Verification items for the finished model (mm, model axes). A direction names the side the tool comes from. Round coordinates to 2 decimals unless told otherwise and drop trailing zeros. Order: outer loops, then holes, each group sorted by start corner. A loop starts at its lowest first (then second) coordinate and runs counter-clockwise, first axis right, second up. Notation, with made-up numbers: M -24,3 L 31,3 A26 cw 31,41 Z; hole C 24.5,34.25 d4. An arc over 180 degrees is marked long. One line per item, written item: value. Start each with the question number.
from build123d import *

# Parameters (mm, degrees)
F3_DEPTH     = 3.5
F4_SIZE      = 1
F5_SIZE      = 0.5
F6_T4_DEPTH  = 8.4221557451
F6_T11_DEPTH = 13.7150489639
F6_T21_DEPTH = 8.4221557451
F6_T28_DEPTH = 8.4221557451
F6_T35_DEPTH = 13.7150489639
F6_T45_DEPTH = 8.4221557451
F7_R         = 1.5
F8_R         = 1
F9_DEPTH     = 25


# Not quite as in the source:
# - a fillet or chamfer that OpenCascade refuses, or shapes differently, is made with other operations: its cross-section is extruded or revolved along the edge and cut away or added


with BuildPart() as f1:
    # F0 (on Front) → F1 (revolve)
    with BuildSketch(Plane.XZ):
        Polygon((0, 7), (0, 0), (5.5, 0), (5.5, 3.5), (6.5, 3.5), (6.5, 7), align=None)
    revolve(axis=Axis((0, 0, 5.0261294236), (0, 0, 1)))

    # F2 (on Front) → F3 (join, symmetric)
    with BuildSketch(Plane.XZ):
        Polygon((3.5, 0), (-3.5, 0), (-3.5, -2.5), (-2, -2.5), (-2, -5.5), (-3.5, -5.5), (-3.5, -7.5), (3.5, -7.5), (3.5, -5.5), (2, -5.5), (2, -2.5), (3.5, -2.5), align=None)
    extrude(amount=F3_DEPTH, both=True)

    # F4
    f4_edges = [f1.edges().sort_by_distance(p)[0] for p in [
        (3.5, -3.5, -1.25),
        (3.5, 3.5, -1.25),
        (-3.5, 3.5, -1.25),
        (-3.5, -3.5, -1.25),
        (-3.5, -3.5, -6.5),
        (3.5, -3.5, -6.5),
        (-3.5, 3.5, -6.5),
        (3.5, 3.5, -6.5),
    ]]
    chamfer(f4_edges, length=F4_SIZE)

    # F5
    f5_edges = [f1.edges().sort_by_distance(p)[0] for p in [
        (2, -3.5, -4),
        (-2, -3.5, -4),
        (-2, 3.5, -4),
        (2, 3.5, -4),
    ]]
    chamfer(f5_edges, length=F5_SIZE)

    # F6: chamfer of 1.5 on 6 edges, made by hand


with BuildPart() as f6_tool2:
    # F6_s3 → F6_t4 (new body)
    with BuildSketch(Plane(origin=(3.7276817198, -3.7276817198, 0), x_dir=(0, 0, 1), z_dir=(-0.7071067812, 0.7071067812, 0))):
        Polygon((-5.5, -5.0355339059), (-4, -3.5355339059), (-5.5, -3.5355339059), align=None)
    extrude(amount=F6_T4_DEPTH)

    split(bisect_by=Plane.XZ.offset(3.5), keep=Keep.BOTTOM)

    split(bisect_by=Plane(origin=(-3, -3, 0), x_dir=(0, 0, 1), z_dir=(0.7071067812, 0.7071067812, 0)), keep=Keep.TOP)

    split(bisect_by=Plane(origin=(1, 0, -1), x_dir=(0, 1, 0), z_dir=(0.7071067812, 0, -0.7071067812)), keep=Keep.TOP)


with BuildPart() as f1_1:
    add(f1.part)

    # F6_t1: union F6_tool2
    add(f6_tool2.part)


with BuildPart() as f6_tool9:
    # F6_s10 → F6_t11 (new body)
    with BuildSketch(Plane.XZ.offset(-6.8575244819)):
        Polygon((-3.5, -5.5), (-2, -4), (-2, -5.5), align=None)
    extrude(amount=F6_T11_DEPTH)

    split(bisect_by=Plane.XZ.offset(3.5), keep=Keep.BOTTOM)

    split(bisect_by=Plane(origin=(-3, -3, 0), x_dir=(0, 0, 1), z_dir=(0.7071067812, 0.7071067812, 0)), keep=Keep.TOP)

    split(bisect_by=Plane.XZ.offset(-3.5), keep=Keep.TOP)

    split(bisect_by=Plane(origin=(-3, 3, 0), x_dir=(0, 0, 1), z_dir=(0.7071067812, -0.7071067812, 0)), keep=Keep.TOP)

    split(bisect_by=Plane(origin=(0.1642135624, -0.1642135624, -0.232233047), x_dir=(0.7071067812, 0.7071067812, 0), z_dir=(0.5, -0.5, -0.7071067812)), keep=Keep.TOP)

    split(bisect_by=Plane(origin=(0.1642135624, 0.1642135624, -0.232233047), x_dir=(-0.7071067812, 0.7071067812, 0), z_dir=(0.5, 0.5, -0.7071067812)), keep=Keep.TOP)


with BuildPart() as f1_2:
    add(f1_1.part)

    # F6_t8: union F6_tool9
    add(f6_tool9.part)


with BuildPart() as f6_tool19:
    # F6_s20 → F6_t21 (new body)
    with BuildSketch(Plane(origin=(3.7276817198, 3.7276817198, 0), x_dir=(0, 0, 1), z_dir=(-0.7071067812, -0.7071067812, 0))):
        Polygon((-5.5, 5.0355339059), (-4, 3.5355339059), (-5.5, 3.5355339059), align=None)
    extrude(amount=F6_T21_DEPTH)

    split(bisect_by=Plane.XZ.offset(-3.5), keep=Keep.TOP)

    split(bisect_by=Plane(origin=(-3, 3, 0), x_dir=(0, 0, 1), z_dir=(0.7071067812, -0.7071067812, 0)), keep=Keep.TOP)

    split(bisect_by=Plane(origin=(1, 0, -1), x_dir=(0, 1, 0), z_dir=(0.7071067812, 0, -0.7071067812)), keep=Keep.TOP)


with BuildPart() as f1_3:
    add(f1_2.part)

    # F6_t18: union F6_tool19
    add(f6_tool19.part)


with BuildPart() as f6_tool26:
    # F6_s27 → F6_t28 (new body)
    with BuildSketch(Plane(origin=(-3.7276817198, -3.7276817198, 0), x_dir=(0, 0, 1), z_dir=(0.7071067812, 0.7071067812, 0))):
        Polygon((-5.5, 5.0355339059), (-4, 3.5355339059), (-5.5, 3.5355339059), align=None)
    extrude(amount=F6_T28_DEPTH)

    split(bisect_by=Plane.XZ.offset(3.5), keep=Keep.BOTTOM)

    split(bisect_by=Plane(origin=(3, -3, 0), x_dir=(0, 0, 1), z_dir=(-0.7071067812, 0.7071067812, 0)), keep=Keep.TOP)

    split(bisect_by=Plane(origin=(-1, 0, -1), x_dir=(0, 1, 0), z_dir=(-0.7071067812, 0, -0.7071067812)), keep=Keep.TOP)


with BuildPart() as f1_4:
    add(f1_3.part)

    # F6_t25: union F6_tool26
    add(f6_tool26.part)


with BuildPart() as f6_tool33:
    # F6_s34 → F6_t35 (new body)
    with BuildSketch(Plane.XZ.offset(-6.8575244819)):
        Polygon((3.5, -5.5), (2, -4), (2, -5.5), align=None)
    extrude(amount=F6_T35_DEPTH)

    split(bisect_by=Plane.XZ.offset(3.5), keep=Keep.BOTTOM)

    split(bisect_by=Plane(origin=(3, -3, 0), x_dir=(0, 0, 1), z_dir=(-0.7071067812, 0.7071067812, 0)), keep=Keep.TOP)

    split(bisect_by=Plane.XZ.offset(-3.5), keep=Keep.TOP)

    split(bisect_by=Plane(origin=(3, 3, 0), x_dir=(0, 0, 1), z_dir=(-0.7071067812, -0.7071067812, 0)), keep=Keep.TOP)

    split(bisect_by=Plane(origin=(-0.1642135624, -0.1642135624, -0.232233047), x_dir=(0.7071067812, -0.7071067812, 0), z_dir=(-0.5, -0.5, -0.7071067812)), keep=Keep.TOP)

    split(bisect_by=Plane(origin=(-0.1642135624, 0.1642135624, -0.232233047), x_dir=(-0.7071067812, -0.7071067812, 0), z_dir=(-0.5, 0.5, -0.7071067812)), keep=Keep.TOP)


with BuildPart() as f1_5:
    add(f1_4.part)

    # F6_t32: union F6_tool33
    add(f6_tool33.part)


with BuildPart() as f6_tool43:
    # F6_s44 → F6_t45 (new body)
    with BuildSketch(Plane(origin=(-3.7276817198, 3.7276817198, 0), x_dir=(0, 0, 1), z_dir=(0.7071067812, -0.7071067812, 0))):
        Polygon((-5.5, -5.0355339059), (-4, -3.5355339059), (-5.5, -3.5355339059), align=None)
    extrude(amount=F6_T45_DEPTH)

    split(bisect_by=Plane.XZ.offset(-3.5), keep=Keep.TOP)

    split(bisect_by=Plane(origin=(3, 3, 0), x_dir=(0, 0, 1), z_dir=(-0.7071067812, -0.7071067812, 0)), keep=Keep.TOP)

    split(bisect_by=Plane(origin=(-1, 0, -1), x_dir=(0, 1, 0), z_dir=(-0.7071067812, 0, -0.7071067812)), keep=Keep.TOP)


with BuildPart() as f1_6:
    add(f1_5.part)

    # F6_t42: union F6_tool43
    add(f6_tool43.part)

    # F7
    f7_edges = [f1_6.edges().sort_by_distance(p)[0] for p in [
        (-6.5, 0, 7),
    ]]
    fillet(f7_edges, radius=F7_R)

    # F8 (on face) → F9 (cut)
    with BuildSketch(Plane(origin=(0, 0, -7.5), x_dir=(1, 0, 0), z_dir=(0, 0, -1))):
        Circle(F8_R)
    extrude(amount=-F9_DEPTH, mode=Mode.SUBTRACT)


solid = f1_6.part
1. Draft check along X on faces 4 (the face through (-0.1, 1.2, 7)), 5 (the face through (-2, 0, -3)), 6 (the face through (0, 1, 0)). Enter one of: released by +X, released by -X, zero draft, split by the parting line, or undercut.
2. Depth check by flat-ended pin: pin 1 (4 mm diameter, centred on y = 4, z = -0.5, fed in from +X); pin 2 (1.2 mm diameter, centred on y = -1, z = -1, fed in from -X); pin 3 (6 mm diameter, centred on x = 0.5, z = -0.5, fed in from -Y). Enter the tip coordinate at first touch or a pass-through.
3. Tool access check on faces 1 (the face through (3, -3, -6)), 2 (the face through (-4, 0, 0)), 3 (the face through (0, 3.5, -4)). Record the directions out of +Z, -Z, +X, -X, +Y, -Y that give a thin tool (end or side, any length) a straight path to the whole face; none if there is none.
4. Section check C-C (z = -1.75). Record the cut outline in (x, y), and give its area (3 significant figures).
5. Scan lines: line 1 along Y through (x, z) = (0, 0.25); line 2 along Y through (x, z) = (0, -1.75); line 3 along Z through (x, y) = (-3, -1.75). Record each from-to range of solid material in increasing order.
6. Section check A-A (x = 0). Record the cut outline in (y, z).
7. Section check B-B (y = 0). Record the cut outline in (x, z), and give its area (3 significant figures).
8. Section check D-D (z = -3.75). Record the cut outline in (x, y), and give its area (3 significant figures).
Geometry check:
1. face 4: zero draft
1. face 5: released by -X
1. face 6: undercut
2. pin 1: stops at x = 5.1
2. pin 2: stops at x = -3.5
2. pin 3: stops at y = -5.5
3. face 1: -Z, +X, -Y
3. face 2: -Z
3. face 3: -Z, +X, -X, +Y
4. outline: M -3.5,-2.5 L -2.5,-3.5 L 2.5,-3.5 L 3.5,-2.5 L 3.5,2.5 L 2.5,3.5 L -2.5,3.5 L -3.5,2.5 Z; hole C 0,0 d2
4. area: 43.9 mm²
5. line 1: y = -5.5 to -1, 1 to 5.5
5. line 2: y = -3.5 to -1, 1 to 3.5
5. line 3: z = -7.5 to -5, -2.5 to 7
6. outline: M -6.5,3.5 L -5.5,3.5 L -5.5,0 L -3.5,0 L -3.5,-7.5 L -1,-7.5 L -1,7 L -5,7 A1.5 ccw -6.5,5.5 Z; M 1,-7.5 L 3.5,-7.5 L 3.5,0 L 5.5,0 L 5.5,3.5 L 6.5,3.5 L 6.5,5.5 A1.5 ccw 5,7 L 1,7 Z
7. outline: M -6.5,3.5 L -5.5,3.5 L -5.5,0 L -3.5,0 L -3.5,-2.5 L -2,-2.5 L -2,-4 L -3.5,-5.5 L -3.5,-7.5 L -1,-7.5 L -1,7 L -5,7 A1.5 ccw -6.5,5.5 Z; M 1,-7.5 L 3.5,-7.5 L 3.5,-5.5 L 2,-4 L 2,-2.5 L 3.5,-2.5 L 3.5,0 L 5.5,0 L 5.5,3.5 L 6.5,3.5 L 6.5,5.5 A1.5 ccw 5,7 L 1,7 Z
7. area: 99.8 mm²
8. outline: M -2,-3 L -1.5,-3.5 L 1.5,-3.5 L 2,-3 L 2,3 L 1.5,3.5 L -1.5,3.5 L -2,3 Z; hole C 0,0 d2
8. area: 24.4 mm²
